Autodesk Inventor part; units mm, degrees
ref_plane "YZ Plane" through (0, 0, 0) normal (1, 0, 0) x (0, 1, 0)
ref_plane "XZ Plane" through (0, 0, 0) normal (0, 1, 0) x (-1, 0, 0)
ref_plane "XY Plane" through (0, 0, 0) normal (0, 0, 1) x (1, 0, 0)
sketch "スケッチ1" plane through (0, 0, 0) normal (0, 0, 1) x (1, 0, 0)
  line L0 (-50, 0) -> (50, 0) construction
  circle A0 centre (-50, 0) radius 4.05
  circle A1 centre (50, 0) radius 4.05
  line L1 (-50, 8.5) -> (50, 8.5)
  line L2 (-50, -8.5) -> (50, -8.5)
  arc A2 (-50, 8.5) -> (-50, -8.5) centre (-50, 0) ccw
  arc A3 (50, -8.5) -> (50, 8.5) centre (50, 0) ccw
  line L3 (55.697, 6.3082) -> (35, 25)
  line L4 (35, 25) -> (-10, 25)
  line L5 (-10, 25) -> (-24.9014, 8.5)
  line L6 (-16.3218, 18) -> (42.751, 18) construction
  line L7 (-10, 25) -> (-10, 18) construction
  line L8 (35, 25) -> (35, 18) construction
  circle A4 centre (32.5, 21.5) radius 1.55
  circle A5 centre (-7.5, 21.5) radius 1.55
  circle A6 centre (12.5, 21.5) radius 1.55
  line L9 (-10, 21.5) -> (35, 21.5) construction
  line L10 (35, 24) -> (-10, 24) construction
  line L11 (-10, 24) -> (-10, 19) construction
  line L12 (-10, 19) -> (35, 19) construction
  line L13 (35, 19) -> (35, 24) construction
  point P0 (0, 0)
  point P1 (0, 0)
  dimension "d0" = 100
  dimension "d1" = 8.1
  dimension "d2" = 8.5
  dimension "d8" = 8.1
  dimension "d10" = 7
  dimension "d11" = 45
  dimension "d12" = 2.5
  dimension "d13" = 3.1
  dimension "d14" = 2.5
  dimension "d15" = 15
  dimension "d17" = 5
  dimension "d18" = 19
extrude "押し出し1" add sketch "スケッチ1" along normal blind 2
fillet "フィレット1" radius 5 3 edges at (-24.9014, 8.5, 1) (-10, 25, 1) (35, 25, 1)
sketch "スケッチ2" plane through (0, 0, 2) normal (0, 0, 1) x (1, 0, 0)
  arc A0 (50, -8.5) -> (55.697, 6.3082) centre (50, 0) ccw
  line L0 (18, -20) -> (-35.4549, -20) construction
  line L1 (-76.9607, -11.5) -> (-72, -11.5)
  line L2 (-72, -11.5) -> (-62, -7)
  line L3 (-62, -7) -> (-32, -7)
  line L4 (-32, -7) -> (-22, -11.5)
  line L5 (-22, -11.5) -> (-17.0393, -11.5)
  line L6 (-17.0393, -11.5) -> (-17.0393, -12.4)
  line L7 (-17.0393, -12.4) -> (-76.9607, -12.4)
  line L8 (-76.9607, -12.4) -> (-76.9607, -11.5)
  line L9 (-31.9893, -6.95) -> (-62.0107, -6.95)
  line L10 (-62.0107, -6.95) -> (-72.0107, -11.45)
  line L11 (-72.0107, -11.45) -> (-77.0107, -11.45)
  line L12 (-77.0107, -11.45) -> (-77.0107, -12.45)
  line L13 (-77.0107, -12.45) -> (-16.9893, -12.45)
  line L14 (-16.9893, -12.45) -> (-16.9893, -11.45)
  line L15 (-16.9893, -11.45) -> (-21.9893, -11.45)
  line L16 (-21.9893, -11.45) -> (-31.9893, -6.95)
  circle A1 centre (-50, 0) radius 4.05
  circle A2 centre (-50, 0) radius 5.5 construction
  circle A3 centre (50, 0) radius 4.05
  line L17 (83.3205, -17.7128) -> (50, 0) construction
  line L18 (50, 0) -> (18, -20) construction
  line L19 (83.3205, -17.7128) -> (37.8533, -17.7128) construction
  line L20 (-11.6402, -10.1128) -> (48.2812, -10.1128)
  line L21 (48.2812, -10.1128) -> (48.2812, -9.2128)
  line L22 (48.2812, -9.2128) -> (43.3205, -9.2128)
  line L23 (43.3205, -9.2128) -> (33.3205, -4.7128)
  line L24 (33.3205, -4.7128) -> (3.3205, -4.7128)
  line L25 (3.3205, -4.7128) -> (-6.6795, -9.2128)
  line L26 (-6.6795, -9.2128) -> (-11.6402, -9.2128)
  line L27 (-11.6402, -9.2128) -> (-11.6402, -10.1128)
  line L28 (-6.6902, -9.1628) -> (3.3098, -4.6628)
  line L29 (3.3098, -4.6628) -> (33.3312, -4.6628)
  line L30 (33.3312, -4.6628) -> (43.3312, -9.1628)
  line L31 (43.3312, -9.1628) -> (48.3312, -9.1628)
  line L32 (48.3312, -9.1628) -> (48.3312, -10.1628)
  line L33 (48.3312, -10.1628) -> (-11.6902, -10.1628)
  line L34 (-11.6902, -10.1628) -> (-11.6902, -9.1628)
  line L35 (-11.6902, -9.1628) -> (-6.6902, -9.1628)
  point P0 (0, 0)
  dimension "d19" = 20
  dimension "d20" = 32
  dimension "d21" = 40
  dimension "d22" = 10
  dimension "d23" = 8.5
  dimension "d24" = 10
  dimension "d25" = 30
  dimension "d26" = 13
  dimension "d27" = 0.05
  dimension "d32" = 11
  dimension "d33" = 120
  dimension "d34" = 1
  dimension "d36" = 5
  dimension "d37" = 40
  dimension "d38" = 8.5
  dimension "d39" = 0.05
extrude "押し出し2" cut sketch "スケッチ2" against normal blind 10 contours L1 L2 L3 L4 L5 L6 L7 L8 | L16 L15 L14 L13 L12 L11 L10 L9 | L27 L26 L25 L24 L23 L22 L21 L20 | L28 L29 L30 L31 L32 L33 L34 L35
fillet "フィレット2" radius 2 7 edges at (-28.5448, -8.5, 1) (-31.9893, -6.95, 1) (-5.2173, -8.5, 1) (3.3098, -4.6628, 1) (41.8583, -8.5, 1) (33.3312, -4.6628, 1) (-54.8936, -6.95, 1)
equation "\"d8\" = d1"
equation "\"d14\" = d12"
equation "\"d24\" = d22"
equation "\"d37\" = d21"
equation "\"d38\" = d23"
properties part number "rinnku" material "GFRP"
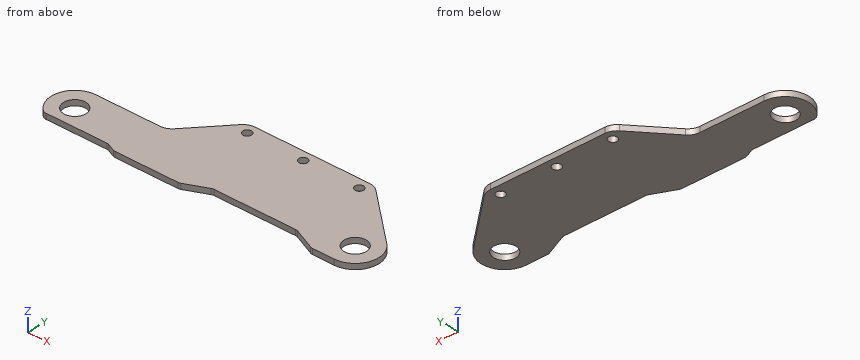
Here's how the part is built. I have some questions about the finished solid (model axes, mm). Give positions to 0.01 mm unless a question says otherwise; leave off trailing zeros. Loops run counter-clockwise (first coordinate to the right, second up) from the corner with the lowest first, then second, coordinate; pieces in that order, holes last. Notation, with made-up numbers: M -14.75,10.25 L 8.25,10.25 A26 cw 8.25,34.25 Z; hole C 54.25,86 d1. An arc over 180 degrees is marked long. Put each result on its own line as item: value. Start each with the question number.
(1) I need wall thicknesses on line 1 along X through (y, z) = (0.5, 0.1); line 2 along X through (y, z) = (3.5, 0.4); line 3 along Y through (x, z) = (-50, 0.95). Which ranges of each line are inside material? Lowest first, please. Write a range as [from, to].
(2) I want a section at B-B on z = 1.15. Please give me the cut outline in (x, y), then the cut area to 3 significant figures.
(3) I want a section at A-A on x = 12.5. Please give me the cut outline in (y, z).
(4) I want a section at C-C on y = 0. Please give me the cut outline in (x, z).
(5) Will these pins go through, and if not, where does the flat tip stop? pin 1 Ø5 at (x, y) = (-50, 0) entering from +Z; pin 2 Ø0.6 at (x, z) = (25.5, 1.5) entering from -Y.
(6) I want a section at D-D on y = 21.5. Please give me the cut outline in (x, z), then the cut area to 3 significant figures.
Answer block:
1. line 1: [-58.49, -54.02], [-45.98, 45.98], [54.02, 58.49]
1. line 2: [-57.75, -52.04], [-47.96, 47.96], [52.04, 57.75]
1. line 3: [-6.95, -4.05], [4.05, 8.5]
2. outline: M -55.51,-6.47 A2 ccw -54.21,-6.95 L -32.42,-6.95 A2 cw -31.6,-7.13 L -28.94,-8.32 A2 ccw -28.12,-8.5 L -5.65,-8.5 A2 ccw -4.83,-8.32 L 2.92,-4.84 A2 cw 3.74,-4.66 L 32.9,-4.66 A2 cw 33.72,-4.84 L 41.47,-8.32 A2 ccw 42.29,-8.5 L 50,-8.5 A8.5 ccw 55.7,6.31 L 36.43,23.71 A5 ccw 33.08,25 L -7.78,25 A5 ccw -11.49,23.35 L -23.41,10.15 A5 cw -27.12,8.5 L -50,8.5 A8.5 ccw Z; hole C -50,0 d8.1; hole C -7.5,21.5 d3.1; hole C 12.5,21.5 d3.1; hole C 32.5,21.5 d3.1; hole C 50,0 d8.1
2. area: 2,630 mm^2
3. outline: M -4.66,0 L 19.95,0 L 19.95,2 L -4.66,2 Z; M 23.05,0 L 25,0 L 25,2 L 23.05,2 Z
4. outline: M -58.5,0 L -54.05,0 L -54.05,2 L -58.5,2 Z; M -45.95,0 L 45.95,0 L 45.95,2 L -45.95,2 Z; M 54.05,0 L 58.5,0 L 58.5,2 L 54.05,2 Z
5. pin 1: through
5. pin 2: y = -4.66
6. outline: M -13.16,0 L -9.05,0 L -9.05,2 L -13.16,2 Z; M -5.95,0 L 10.95,0 L 10.95,2 L -5.95,2 Z; M 14.05,0 L 30.95,0 L 30.95,2 L 14.05,2 Z; M 34.05,0 L 38.88,0 L 38.88,2 L 34.05,2 Z
6. area: 85.5 mm^2
